Verification items for this drawing (mm, ordinates from the low corner). A direction names the side the tool comes from. Give positions to 0.01 mm unless a question says otherwise; leave off trailing zeros. Loops run counter-clockwise (first coordinate to the right, second up) from the corner with the lowest first, then second, coordinate; pieces in that order, holes last. Notation, with made-up numbers: (66.5, 81) -> (77.5, 81) arc R24 cw to (77.5, 112) -> close; hole circle Ø10 at (77.25, 11.5). An arc over 180 degrees is marked (long way). Write item = value, one per line.
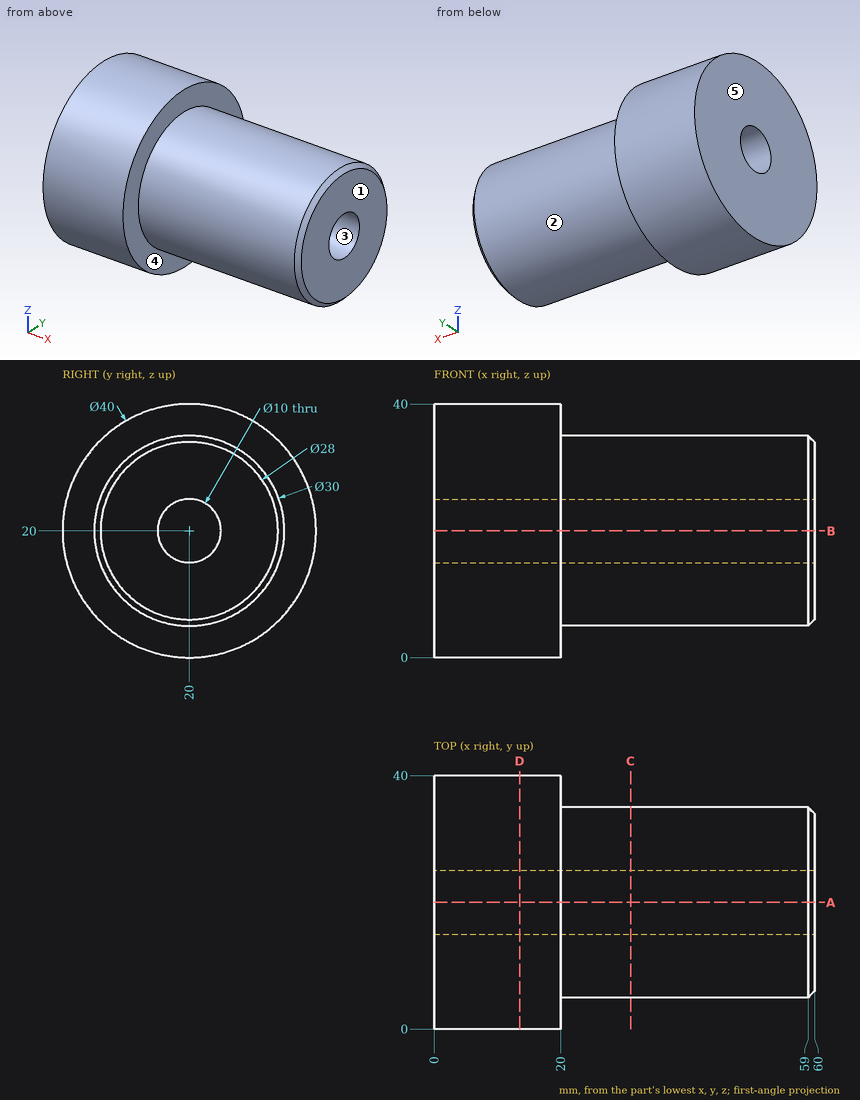
Item 1: Draft check along Y on the marked faces 1, 2 and 3. Enter one of: +Y half, -Y half, draft (parallel to the pull), parting line (faces both ways), or undercut.
Answer:
face_1 = draft
face_2 = parting line
face_3 = undercut
Item 2: Thickness scan on L1, parallel to Z at x = 17, y = 20; L2, parallel to Z at x = 32, y = 20; L3, parallel to X at y = 4.5, z = 27. Record the ranges inside material, lowest first. Write a range as [from, to].
Answer:
L1 = [0, 15], [25, 40]
L2 = [5, 15], [25, 35]
L3 = [0, 20]
Item 3: Section check A-A, the plane y = 20. Record the cut outline in (x, z), plus the area to 3 significant figures.
Answer:
outline = (0, 0) -> (20, 0) -> (20, 5) -> (59, 5) -> (60, 6) -> (60, 15) -> (0, 15) -> close; (0, 25) -> (60, 25) -> (60, 34) -> (59, 35) -> (20, 35) -> (20, 40) -> (0, 40) -> close
area = 1,400 mm^2
Item 4: Section check D-D, the plane x = 13.5. Record the cut outline in (y, z), plus the area to 3 significant figures.
Answer:
outline = circle Ø40 at (20, 20); hole circle Ø10 at (20, 20)
area = 1,180 mm^2
Item 5: Section check C-C, the plane x = 31. Record the cut outline in (y, z).
Answer:
outline = circle Ø30 at (20, 20); hole circle Ø10 at (20, 20)
Item 6: Gauge pin test, flat ends, axial feed: pin 1 (1.5 mm diameter, centred on x = 31.5, z = 7.5, fed in from -Y); pin 2 (3 mm diameter, centred on x = 12, y = 8, fed in from +Z); pin 3 (1 mm diameter, centred on x = 8.5, z = 25, fed in from -Y); pin 4 (2 mm diameter, centred on y = 17.5, z = 22.5, fed in from -X). Record the tip position at first contact, or that the pin passes through.
Answer:
pin_1 = 10.68
pin_2 = 37.02
pin_3 = 0.51
pin_4 = through
Item 7: Tool access check on the marked faces 4 and 5. Record the directions out of +Z, -Z, +X, -X, +Y, -Y that give a thin tool (end or side, any length) a straight path to the whole face; none if there is none.
Answer:
face_4 = +X
face_5 = +Z, -Z, -X, +Y, -Y
